Build history of the part. All positions in model axes, mm. A direction names the side the tool comes from. Give positions to 0.01 mm unless a question says otherwise; leave off trailing zeros. Order: outer loops, then holes, each group sorted by start corner. A loop starts at its lowest first (then second) coordinate and runs counter-clockwise, first axis right, second up. Notation, with made-up numbers: (19, 16.25) - (53, 16.25) arc R18 ccw to (53, 23.25) - close; hole circle Ø5 at (32, 12). An arc over 180 degrees is marked (long way). Use a Markdown table: item, result. Add a question column.
(1) Slice it at B-B (x = 46). Write the cut outline in (y, z).
(2) Flat gauge pins, fed straight in: pin 1 (1.3 mm diameter, centred on y = 4, z = 69, fed in from +X); pin 2 (4 mm diameter, centred on y = 9.52, z = 60.48, fed in from +X); pin 3 (4 mm diameter, centred on y = 4.89, z = 52.15, fed in from -X). Where does each tip first touch, or does it go through?
(3) Wall check: line 1 (Y direction, x = -10, z = 60). Give the ranges that are in metal, low to high.
(4) Slice it at A-A (y = 0). Write the cut outline in (x, z) (3 decimals), then the cut area to 3 significant figures.
(5) Which spindle directions (+Z, -Z, +X, -X, +Y, -Y) get a long thin tool onto all of the face, cutting with end or side? Do faces 1 (the face through (-61.5, -10, 62)), 2 (the face through (-57.15, -1, 53)), 3 (the face through (62.51, 8.66, 58.4)). Say none if no direction does.
(6) Mould opens along Y. For faces 4 (the face through (59.3, -4.8, 66.9)), 5 (the face through (-1, 63.5, 60)) say: +Y half, -Y half, draft (parallel to the pull), parting line (faces both ways), or undercut.
from build123d import *

# Parameters (mm, degrees)
BOSS_EXTRUDE1_DEPTH            = 76.2
BOSS_EXTRUDE1_DEPTH_BACK       = 76.2
SKETCH3_W                      = 127
SKETCH3_H                      = 127
SKETCH3_W_2                    = 114.3
SKETCH3_H_2                    = 114.3
SKETCH6_W                      = 127
SKETCH6_H                      = 120.65
CUT_EXTRUDE1_DEPTH             = 162.144934764
M12_CLEARANCE_HOLE1_D          = 13.5
CBORE_FOR_M3_SHCS1_D           = 3.2
CBORE_FOR_M3_SHCS1_DEPTH       = 6.35
CBORE_FOR_M3_SHCS1_CBORE_D     = 4.5
CBORE_FOR_M3_SHCS1_CBORE_DEPTH = 2
CBORE_FOR_M3_SHCS2_D           = 3.2
CBORE_FOR_M3_SHCS2_CBORE_D     = 4.5
CBORE_FOR_M3_SHCS2_CBORE_DEPTH = 2


with BuildPart() as part:
    # Sketch3 → Boss-Extrude1 (new, two sides: drawn at the far end of the back side and taken through both)
    with BuildSketch(Plane.XY.offset(-BOSS_EXTRUDE1_DEPTH_BACK)):
        Rectangle(SKETCH3_W, SKETCH3_H)
        Rectangle(SKETCH3_W_2, SKETCH3_H_2, mode=Mode.SUBTRACT)
    extrude(amount=BOSS_EXTRUDE1_DEPTH + BOSS_EXTRUDE1_DEPTH_BACK)

    # Sketch6 → Cut-Extrude1 (cut, through all)
    with BuildSketch(Plane(origin=(0, 63.5, 0), x_dir=(1, 0, 0), z_dir=(0, 1, 0))):
        with Locations((0, 15.875)):
            Rectangle(SKETCH6_W, SKETCH6_H)
    extrude(amount=-CUT_EXTRUDE1_DEPTH, mode=Mode.SUBTRACT)

    # M12 Clearance Hole1 (through all)
    with Locations(Plane(origin=(63.5, 0, 0), x_dir=(0, 0, -1), z_dir=(1, 0, 0))):
        with Locations((-60.325, 0)):
            Hole(M12_CLEARANCE_HOLE1_D / 2)

    # CBORE for M3 SHCS1
    with Locations(Plane(origin=(63.5, 0, 0), x_dir=(0, 0, -1), z_dir=(1, 0, 0))):
        with Locations((-68.496426866, -4.894221897), (-68.649233927, 4.629552303), (-60.477807061, 9.523774199), (-52.153573134, 4.894221897), (-52.000766073, -4.629552303), (-60.172192939, -9.523774199)):
            CounterBoreHole(CBORE_FOR_M3_SHCS1_D / 2, CBORE_FOR_M3_SHCS1_CBORE_D / 2, CBORE_FOR_M3_SHCS1_CBORE_DEPTH, depth=CBORE_FOR_M3_SHCS1_DEPTH)

    # CBORE for M3 SHCS2 (through all)
    with Locations(Plane.ZY.offset(63.5)):
        with Locations((68.649233927, 4.629552303), (60.477807061, 9.523774199), (68.496426866, -4.894221897), (52.153573134, 4.894221897), (52.000766073, -4.629552303), (60.172192939, -9.523774199)):
            CounterBoreHole(CBORE_FOR_M3_SHCS2_D / 2, CBORE_FOR_M3_SHCS2_CBORE_D / 2, CBORE_FOR_M3_SHCS2_CBORE_DEPTH)


solid = part.part
Solution:
| question | item | result |
|---|---|---|
| 1 | outline | (-63.5, 44.45) - (-57.15, 44.45) - (-57.15, 76.2) - (-63.5, 76.2) - close; (57.15, 44.45) - (63.5, 44.45) - (63.5, 76.2) - (57.15, 76.2) - close |
| 2 | pin 1 | through |
| 2 | pin 2 | x = 61.5 |
| 2 | pin 3 | x = -61.5 |
| 3 | line 1 | -63.5 to -57.15, 57.15 to 63.5 |
| 4 | outline | (-63.5, 44.45) - (-57.15, 44.45) - (-57.15, 53.575) - (-63.5, 53.575) - close; (-63.5, 67.075) - (-57.15, 67.075) - (-57.15, 76.2) - (-63.5, 76.2) - close; (57.15, 44.45) - (63.5, 44.45) - (63.5, 53.575) - (57.15, 53.575) - close; (57.15, 67.075) - (63.5, 67.075) - (63.5, 76.2) - (57.15, 76.2) - close |
| 4 | area | 232 mm2 |
| 5 | face 1 | -X |
| 5 | face 2 | +Z, -Z |
| 5 | face 3 | +X |
| 6 | face 4 | undercut |
| 6 | face 5 | +Y half |
